The model under review builds one solid part; all positions refer to its coordinate system, in mm. A direction names the side the tool comes from. Round coordinates to 2 decimals unless told otherwise and drop trailing zeros. Order: outer loops, then holes, each group sorted by start corner. A loop starts at its lowest first (then second) coordinate and runs counter-clockwise, first axis right, second up. Notation, with made-up numbers: (-4.5, -37) -> (43.5, -37) arc R24 ccw to (43.5, 0) -> close; hole circle Ø1 at (31.25, 17.25). An arc over 180 degrees is marked (long way). Use a Markdown table: item, result. Add a question column.
```python
from build123d import *

# Parameters (mm, degrees)
BOSS_EXTRUDE1_DEPTH = 60
SKETCH2_W           = 50
SKETCH2_H           = 27.071067812
CUT_EXTRUDE1_DEPTH  = 50
FILLET1_R           = 10
CHAMFER1_SIZE       = 2
SKETCH3_R           = 2
CUT_EXTRUDE2_DEPTH  = 30
CHAMFER2_SIZE       = 5
CHAMFER2_SIZE2      = 3.535533906


with BuildPart() as part:
    # Sketch1 → Boss-Extrude1 (new body)
    with BuildSketch(Plane.XY):
        Polygon((0, 0), (-60, 0), (-60, 27.071067812), (-44.393398282, 42.67766953), (-40.857864376, 39.142135624), (-55, 25), (-55, 5), (0, 5), align=None)
    extrude(amount=BOSS_EXTRUDE1_DEPTH)

    # Sketch2 → Cut-Extrude1 (cut)
    with BuildSketch(Plane.ZY.offset(60)):
        with Locations((30, 13.535533906)):
            Rectangle(SKETCH2_W, SKETCH2_H)
    extrude(amount=-CUT_EXTRUDE1_DEPTH, mode=Mode.SUBTRACT)

    # Fillet1
    fillet1_edges = [part.edges().sort_by_distance(p)[0] for p in [
        (0, 2.5, 60),
        (-55, 5, 57.5),
        (-60, 0, 57.5),
        (-42.625631329, 40.909902577, 60),
        (-55, 5, 2.5),
        (-60, 0, 2.5),
        (-10, 2.5, 5),
        (-10, 2.5, 55),
        (-42.625631329, 40.909902577, 0),
        (0, 2.5, 0),
    ]]
    fillet(fillet1_edges, radius=FILLET1_R)

    # Chamfer1
    chamfer1_edges = [part.edges().sort_by_distance(p)[0] for p in [
        (-55, 20, 5),
        (-10, 5, 30),
        (-32.5, 5, 5),
        (-55, 20, 55),
        (-32.5, 5, 55),
        (-55, 20, 0),
        (-27.5, 5, 0),
        (-27.5, 5, 60),
        (-55, 20, 60),
        (0, 5, 30),
        (-2.928932188, 5, 57.071067812),
        (-2.928932188, 5, 2.928932188),
        (-12.928932188, 5, 7.928932188),
        (-12.928932188, 5, 52.071067812),
        (-52.071067812, 7.928932188, 0),
        (-52.071067812, 7.928932188, 5),
        (-52.071067812, 7.928932188, 55),
        (-52.071067812, 7.928932188, 60),
    ]]
    chamfer(chamfer1_edges, length=CHAMFER1_SIZE)

    # Sketch3 → Cut-Extrude2 (cut)
    with BuildSketch(Plane(origin=(-43.535533906, 43.535533906, 0), x_dir=(0, 0, 1), z_dir=(-0.7071067811865464, 0.7071067811865488, 0))):
        with Locations(Location((30, -6.284271247, 0), (0, 0, 270))):
            Circle(SKETCH3_R)
        with Locations(Location((36, -12.284271247, 0), (0, 0, 270))):
            Circle(SKETCH3_R)
        with Locations(Location((24, -12.284271247, 0), (0, 0, 270))):
            Circle(SKETCH3_R)
        with Locations(Location((18, -6.284271247, 0), (0, 0, 270))):
            Circle(SKETCH3_R)
        with Locations(Location((12, -12.284271247, 0), (0, 0, 270))):
            Circle(SKETCH3_R)
        with Locations(Location((42, -6.284271247, 0), (0, 0, 270))):
            Circle(SKETCH3_R)
        with Locations(Location((48, -12.284271247, 0), (0, 0, 270))):
            Circle(SKETCH3_R)
    extrude(amount=-CUT_EXTRUDE2_DEPTH, mode=Mode.SUBTRACT)

    # Chamfer2
    chamfer2_edges = [part.edges().sort_by_distance(p)[0] for p in [
        (-60, 27.071067812, 30),
    ]]
    chamfer2_side = [part.faces().sort_by_distance(p)[0] for p in [
        (-52.552716381, 34.518351431, 30),
    ]]
    chamfer(chamfer2_edges, length=CHAMFER2_SIZE, length2=CHAMFER2_SIZE2, reference=chamfer2_side[0])


solid = part.part
```
Q1. Add section B-B, the plane z = 21. Give the boundary of the cut face in (x, y).
Q2. For faces 5 (the face through (-55, 27.071, 30)), 6 (the face through (-56, 20, 56)), 7 (the face through (-12.61, 3.57, 7.44)), 8 (the face through (-52.536, 7.628, 1.458)), 9 (the face through (-10, 2, 30)), list the 3-axis set-ups (+Z, -Z, +X, -X, +Y, -Y) from which the entire face can be reached by the end or side of a thin tool; tool diameter is ignored.
Q3. Add section A-A, the plane x = -37.5. Give the boundary of the cut face in (y, z), then the cut area to 3 significant figures.
Q4. To check wall thickness, follow line 1 along Z through (x, y) = (-23.5, 4); line 2 along Y through (x, z) = (-55.5, 25.5); line 3 along X through (y, z) = (35.5, 11). State the ranges of each line that lie inside material, in increasing order.
Q5. For pin 1 (3 mm diameter, centred on y = 29, z = 24.5, fed in from -X); pin 2 (12 mm diameter, centred on x = -53, z = 36.5, fed in from -Y); pin 3 (8 mm diameter, centred on x = -17, z = 30, fed in from -Y); pin 4 (1.5 mm diameter, centred on y = 1.5, z = 23, fed in from -X), all flat-tipped, find the tip position at first contact; note any pin that passes through.
Q6. Draft analysis for pull direction Z (two halves, no side actions). For faces 1 (the face through (-28, 4, 1)), 2 (the face through (-52.372, 7.464, 56.458)), 3 (the face through (-56.464, 29, 30)), 4 (the face through (-51.99, 7.85, 57.51)), state which applies: released by +Z, released by -Z, zero draft, split by the parting line, or undercut.
Return value:
| question | item | result |
|---|---|---|
| 1 | outline | (-56.46, 27.07) -> (-52.93, 27.07) -> (-40.86, 39.14) -> (-44.39, 42.68) -> (-56.46, 30.61) -> close; (-10, 0) -> (0, 0) -> (0, 3) -> (-2, 5) -> (-8, 5) -> (-10, 3) -> close |
| 2 | face 5 | +X, -X, -Y |
| 2 | face 6 | +X |
| 2 | face 7 | +Y |
| 2 | face 8 | -Z, +X |
| 2 | face 9 | -X, +Y, -Y |
| 3 | outline | (0, 0) -> (3, 0) -> (5, 2) -> (5, 3) -> (3, 5) -> (0, 5) -> close; (0, 55) -> (3, 55) -> (5, 57) -> (5, 58) -> (3, 60) -> (0, 60) -> close |
| 3 | area | 42.0 mm² |
| 4 | line 1 | 1 to 4, 56 to 59 |
| 4 | line 2 | 27.07 to 31.57 |
| 4 | line 3 | -50.42 to -44.5 |
| 5 | pin 1 | x = -56.46 |
| 5 | pin 2 | y = 27.07 |
| 5 | pin 3 | through |
| 5 | pin 4 | x = -10 |
| 6 | face 1 | released by -Z |
| 6 | face 2 | undercut |
| 6 | face 3 | undercut |
| 6 | face 4 | zero draft |
